```python
from build123d import *

# Parameters (mm, degrees)
SKETCH2_R           = 8.5
SKETCH2_R_2         = 7
BOSS_EXTRUDE1_DEPTH = 0.8
CUT_EXTRUDE1_DEPTH  = 13.04740636
CIRPATTERN2_COUNT   = 19


with BuildPart() as part:
    # Sketch2 → Boss-Extrude1 (new body)
    with BuildSketch(Plane.XY):
        Circle(SKETCH2_R)
        Circle(SKETCH2_R_2, mode=Mode.SUBTRACT)
    extrude(amount=BOSS_EXTRUDE1_DEPTH)

    # Sketch3 → Cut-Extrude1 (cut, symmetric)
    with BuildSketch(Plane.XY):
        with BuildLine():
            Line((21.193331558, 54.843524577), (3.301793839, 7.83250646))
            ThreePointArc((3.301793839, 7.83250646), (2.547786774, 7.478098476), (2.166996346, 8.219131757))
            Line((2.166996346, 8.219131757), (16.698741556, 56.374830563))
            Line((16.698741556, 56.374830563), (49.142224258, 151.600836547))
            Line((49.142224258, 151.600836547), (53.63681426, 150.069530561))
            Line((53.63681426, 150.069530561), (21.193331558, 54.843524577))
        make_face()
    cut_extrude1 = extrude(amount=CUT_EXTRUDE1_DEPTH, both=True, mode=Mode.SUBTRACT)

    # CirPattern2: Cut-Extrude1 ×19 about axis
    cirpattern2_axis = Axis((0, 0, 0), (0, 0, 1))
    for i in range(1, CIRPATTERN2_COUNT):
        add(cut_extrude1.rotate(cirpattern2_axis, i * 360 / CIRPATTERN2_COUNT), mode=Mode.SUBTRACT)


solid = part.part
```
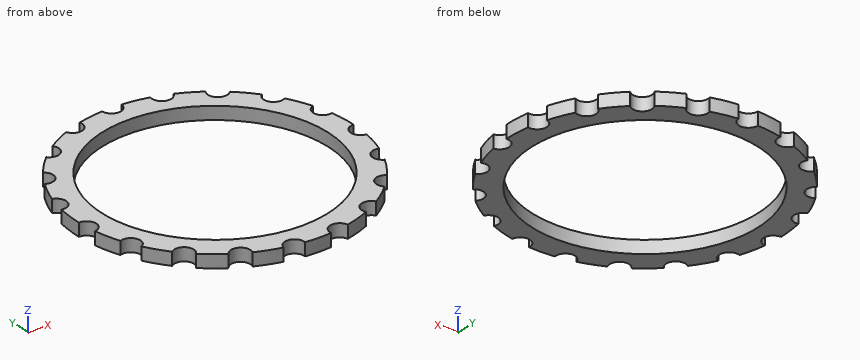
Can you work these out from the model? Positions are in its coordinate system, mm. Round coordinates to 2 decimals unless told otherwise and drop trailing zeros. Loops run counter-clockwise (first coordinate to the right, second up) from the corner with the lowest first, then second, coordinate; pieces in that order, holes last. Notation, with made-up numbers: M 17.25,-23.75 L 31.25,-23.75 A30 ccw 31.25,-1.75 Z; hole C -37,-11 d2. An arc over 180 degrees is marked long. Answer as a JSON object with one key per item and string values. Group by question number.
Q1. Imagine slicing it at C-C, the plane y = -7.5. Please give me the cut outline in (x, z).
Q2. Please list where these lines run through material, in increasing order: L1, parallel to Y at x = 0, z = 0.45; L2, parallel to X at y = -1.5, z = 0.6; L3, parallel to Y at x = 2.25, z = 0.2.
Q3. Imagine slicing it at A-A, the plane x = -1.5. Please give me the cut outline in (y, z).
Q4. Imagine slicing it at B-B, the plane y = 5.5. Please give me the cut outline in (x, z), then the cut area to 3 significant figures.
Q5. Will this pin go through, and if not, where does the flat tip stop? pin 1 (6 mm diameter, centred on x = 5.5, y = -1.5, fed in from -Z).
Findings:
{
 "1": {"outline": "M -3.43,0 L 3.46,0 L 3.46,0.8 L -3.43,0.8 Z"},
 "2": {"L1": "y = -8.5 to -7, 7 to 7.9", "L2": "x = -8.37 to -6.84, 6.84 to 8.37", "L3": "y = -8.2 to -6.63, 6.63 to 7.7"},
 "3": {"outline": "M -7.8,0 L -6.84,0 L -6.84,0.8 L -7.8,0.8 Z; M 6.84,0 L 8.37,0 L 8.37,0.8 L 6.84,0.8 Z"},
 "4": {"outline": "M -6.48,0 L -4.33,0 L -4.33,0.8 L -6.48,0.8 Z; M 4.33,0 L 6.48,0 L 6.48,0.8 L 4.33,0.8 Z", "area": "3.44 mm2"},
 "5": {"pin 1": "stops at z = 0"}
}
